```python
from build123d import *

# Parameters (mm, degrees)
BOSS_EXTRUDE1_DEPTH = 210
BOSS_EXTRUDE2_DEPTH = 100
SKETCH3_R           = 2.75
CUT_EXTRUDE1_DEPTH  = 20
FILLET1_R           = 5


with BuildPart() as part:
    # Sketch1 → Boss-Extrude1 (new body)
    with BuildSketch(Plane(origin=(0, 0, 0), x_dir=(0, 0, -1), z_dir=(1, 0, 0))):
        Polygon((0, 0), (0, 120), (-8, 120), (-8, 8), (-180, 8), (-180, 0), align=None)
    extrude(amount=BOSS_EXTRUDE1_DEPTH)

    # Sketch2 → Boss-Extrude2 (add)
    with BuildSketch(Plane(origin=(0, 8, 0), x_dir=(1, 0, 0), z_dir=(0, 1, 0))):
        Polygon((5, -8), (5, -175), (205, -175), (205, -8), (210, -8), (210, -180), (0, -180), (0, -8), align=None)
    extrude(amount=BOSS_EXTRUDE2_DEPTH)

    # Sketch3 → Cut-Extrude1 (cut)
    with BuildSketch(Plane.XZ):
        with Locations(Location((24, 140, 0), (0, 0, 270))):
            Circle(SKETCH3_R)
        with Locations(Location((81, 140, 0), (0, 0, 270))):
            Circle(SKETCH3_R)
        with Locations(Location((186, 140, 0), (0, 0, 270))):
            Circle(SKETCH3_R)
        with Locations(Location((129, 140, 0), (0, 0, 270))):
            Circle(SKETCH3_R)
    extrude(amount=-CUT_EXTRUDE1_DEPTH, mode=Mode.SUBTRACT)

    # Fillet1
    fillet1_edges = [part.edges().sort_by_distance(p)[0] for p in [
        (210, 54, 180),
        (205, 58, 175),
        (5, 58, 175),
        (0, 54, 180),
    ]]
    fillet(fillet1_edges, radius=FILLET1_R)


solid = part.part
```
Geometry check sheet. Reference: the model listing, model coordinates, mm. A direction names the side the tool comes from. Coordinates: 2 decimals unless noted, no trailing zeros. Loops run counter-clockwise (first coordinate to the right, second up) from the corner with the lowest first, then second, coordinate; pieces in that order, holes last.
Item 1: Sectioned sample at B-B, the plane z = 140. Record the boundary of the cut face in (x, y), then the cut area to 3 significant figures.
Item 2: Go/stop test with flat-tipped pins: pin 1 Ø5 at (x, z) = (129, 140) entering from -Y; pin 2 Ø7 at (x, z) = (186, 140) entering from +Y. Record where each tip stops, or that it passes through.
Item 3: Access from +Z, -Z, +X, -X, +Y, -Y to the whole of each face (thin tool, end or side, straight path). Record for faces 1 (the face through (104, 59, 0)), 2 (the face through (104, 57, 175)), 3 (the face through (105, 108, 176)).
Item 4: Thickness scan on line 1 (X direction, y = 4, z = 140); line 2 (X direction, y = 53, z = 45.5); line 3 (Z direction, x = 55, y = 69). Record the ranges inside material, lowest first.
Item 5: Sectioned sample at A-A, the plane x = 129. Record the boundary of the cut face in (y, z), then the cut area to 3 significant figures.
Item 6: Release check for a two-part mould opening along Z. For faces 4 (the face through (81.83, 3.94, 137.38)), 5 (the face through (1, 55, 178)), 6 (the face through (0, 61, 89)) record: released by +Z, released by -Z, zero draft, split by the parting line, or undercut.
Item 7: Sectioned sample at C-C, the plane y = 56. Record the boundary of the cut face in (x, z), then the cut area to 3 significant figures.
Item 8: Sectioned sample at D-D, the plane x = 180.5. Record the boundary of the cut face in (y, z).
Check result:
1. outline: (0, 0) - (21.25, 0) - (21.25, 8) - (5, 8) - (5, 108) - (0, 108) - close; (26.75, 0) - (78.25, 0) - (78.25, 8) - (26.75, 8) - close; (83.75, 0) - (126.25, 0) - (126.25, 8) - (83.75, 8) - close; (131.75, 0) - (183.25, 0) - (183.25, 8) - (131.75, 8) - close; (188.75, 0) - (210, 0) - (210, 108) - (205, 108) - (205, 8) - (188.75, 8) - close
1. area: 2,500 mm2
2. pin 1: passes through
2. pin 2: stops at y = 8
3. face 1: -Z, +X, -X, +Y, -Y
3. face 2: +Y
3. face 3: +Z, +X, -X, +Y
4. line 1: x = 0 to 21.25, 26.75 to 78.25, 83.75 to 126.25, 131.75 to 183.25, 188.75 to 210
4. line 2: x = 0 to 5, 205 to 210
4. line 3: z = 0 to 8, 175 to 180
5. outline: (0, 0) - (120, 0) - (120, 8) - (8, 8) - (8, 137.25) - (0, 137.25) - close; (0, 142.75) - (8, 142.75) - (8, 175) - (108, 175) - (108, 180) - (0, 180) - close
5. area: 2,790 mm2
6. face 4: undercut
6. face 5: released by +Z
6. face 6: zero draft
7. outline: (0, 0) - (210, 0) - (210, 175) arc R5 ccw to (205, 180) - (5, 180) arc R5 ccw to (0, 175) - close; hole (5, 8) - (205, 8) - (205, 170) arc R5 ccw to (200, 175) - (10, 175) arc R5 ccw to (5, 170) - close
7. area: 4,400 mm2
8. outline: (0, 0) - (120, 0) - (120, 8) - (8, 8) - (8, 175) - (108, 175) - (108, 180) - (0, 180) - close
